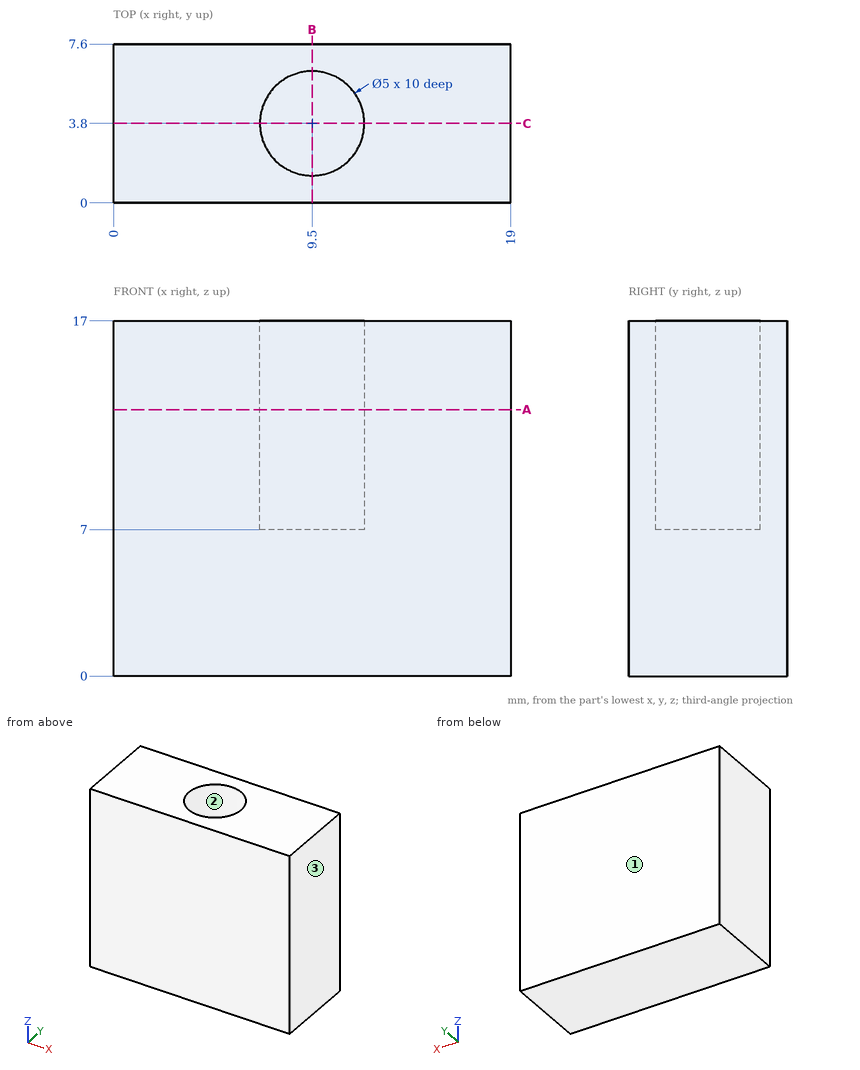
Can you work these out from the drawing? Everything is in mm from the part's minimum corner. Round coordinates to 2 decimals unless told otherwise and drop trailing zeros. Loops run counter-clockwise (first coordinate to the right, second up) from the corner with the lowest first, then second, coordinate; pieces in that order, holes last. Notation, with made-up numbers: (7.5, 35) - (16.5, 35) arc R13 cw to (16.5, 51) - close; hole circle Ø11 at (-13, -18.75). An arc over 180 degrees is marked (long way). Answer in a Markdown table with one row per item. Add a question column.
(1) I'm going to push a flat-ended pin straight in: pin 1 (1.5 mm diameter, centred on x = 10.5, y = 4.5, fed in from +Z). Where does the tip first touch, or does it pass through?
(2) If we section it at A-A (z = 12.75): Please give me the cut outline in (x, y), plus the area to 3 significant figures.
(3) If we section it at C-C (y = 3.8): Please give me the cut outline in (x, z).
(4) I need wall thicknesses on line 1 along Y through (x, z) = (9.5, 10); line 2 along Z through (x, y) = (9.25, 4.5); line 3 along Y through (x, z) = (10, 14.5). Which ranges of each line are inside material? Lowest first, please.
(5) If we mould it in two halves opening along Y, with no side actions, what happens to the marked faces 1, 2 and 3? For each: pulls with the +Y half, pulls with the -Y half, needs draft (parallel to the pull), parting line crosses it, or undercut.
(6) If we section it at B-B (x = 9.5): Please give me the cut outline in (y, z), plus the area to 3 significant figures.
Model answer:
| question | item | result |
|---|---|---|
| 1 | pin 1 | stops at z = 7 |
| 2 | outline | (0, 0) - (19, 0) - (19, 7.6) - (0, 7.6) - close; hole circle Ø5 at (9.5, 3.8) |
| 2 | area | 125 mm² |
| 3 | outline | (0, 0) - (19, 0) - (19, 17) - (12, 17) - (12, 7) - (7, 7) - (7, 17) - (0, 17) - close |
| 4 | line 1 | y = 0 to 1.3, 6.3 to 7.6 |
| 4 | line 2 | z = 0 to 7 |
| 4 | line 3 | y = 0 to 1.35, 6.25 to 7.6 |
| 5 | face 1 | pulls with the +Y half |
| 5 | face 2 | undercut |
| 5 | face 3 | needs draft |
| 6 | outline | (0, 0) - (7.6, 0) - (7.6, 17) - (6.3, 17) - (6.3, 7) - (1.3, 7) - (1.3, 17) - (0, 17) - close |
| 6 | area | 79.2 mm² |
